Here's how the part is built. I have some questions about the finished solid (model axes, mm). Face numbers are marked on the shaded views. A direction names the side the tool comes from. Coordinates: 2 decimals unless noted, no trailing zeros. Write each loop counter-clockwise with the first axis right and the second up, starting at its lowest first coordinate (ties: lowest second). Pieces come first, ordered by that corner, then holes.
Item 1: If I drill on line 1 (X direction, y = -4.5, z = -3.75); line 2 (Y direction, x = -10, z = -9.5); line 3 (X direction, y = -2, z = -3.75), over which ranges is the centre line in solid material (lowest first)?
Item 2: If we section it at B-B (x = 0): Please give me the cut outline in (y, z).
Item 3: For the marked faces 5 and 6, which set-ups out of +Z, -Z, +X, -X, +Y, -Y let a thin tool reach every point of the face, with its end or its side?
Item 4: If we section it at A-A (z = -1): Please give me the cut outline in (x, y), then the cut area to 3 significant figures.
Item 5: I'm going to push flat-ended pins straight in: pin 1 Ø2.5 at (x, z) = (-6, -3) entering from +Y; pin 2 Ø4 at (x, y) = (0.03, -11.5) entering from -Z; pin 3 Ø5 at (x, y) = (-9.97, 5.73) entering from +Z; pin 4 Ø1.5 at (y, z) = (-4, -5) entering from -X. Where does each tip first touch, or does it pass through?
Item 6: If we section it at C-C (y = -11.5): Please give me the cut outline in (x, z).
Item 7: If we section it at D-D (x = 9): Please give me the cut outline in (y, z), then the cut area to 3 significant figures.
Item 8: We'd pull the mould along Y, two halves only. Please class the marked faces 1, 2, 3 and 4: +Y half, -Y half, draft (parallel to the pull), parting line (faces both ways), or undercut.
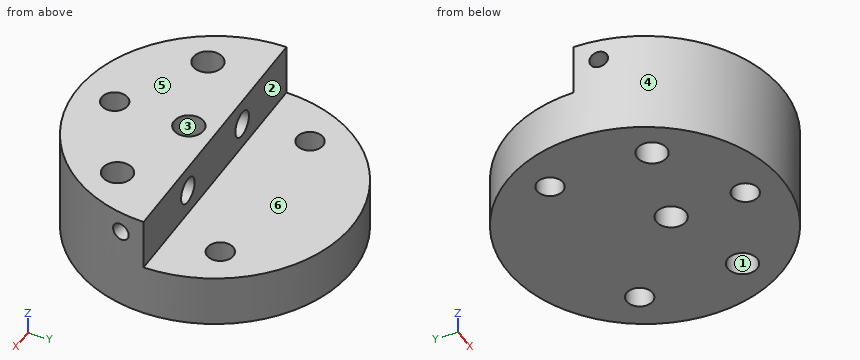
Autodesk Inventor part; units mm, degrees
ref_plane "作業平面8" through (15.56, -2.7436, 0) normal (0.9848, -0.1736, 0) x (0, 0, 1)
ref_plane "作業平面9" through (-15.56, -2.7436, 0) normal (0.9848, 0.1736, 0) x (0, 0, 1)
ref_plane "XZ Plane" through (0, 0, 0) normal (0, 1, 0) x (-1, 0, 0)
sketch "スケッチ2" plane through (0, 0, 0) normal (0, 0, 1) x (1, 0, 0)
  circle A0 centre (0, 0) radius 15.8
  dimension "d0" = 31.6
extrude "押し出し1" add sketch "スケッチ2" against normal blind 12
sketch "スケッチ4" plane through (0, 0, 0) normal (0, 0, 1) x (1, 0, 0)
  circle A0 centre (0.0258, -11.5) radius 1.5
  circle A1 centre (9.9464, 5.7723) radius 1.5
  circle A2 centre (-9.9722, 5.7277) radius 1.5
  point P0 (0, 0)
  dimension "d8" = 3
  dimension "d9" = 11.5
  dimension "d12" = 360
extrude "押し出し3" cut sketch "スケッチ4" against normal through all
sketch "スケッチ13" plane through (0, 0, 0) normal (0, 0, 1) x (1, 0, 0)
  circle A0 centre (-10, -6) radius 1.7
  circle A1 centre (10, -6) radius 1.7
  circle A2 centre (0, -3) radius 1.7
  line L0 (0, 0) -> (0, -19.4065)
  line L1 (0, 0) -> (20.4623, 0)
  point P0 (0, -4.7)
  point P1 (0, -1.3)
  dimension "d125" = 3.4
  dimension "d126" = 3.4
  dimension "d127" = 3.4
  dimension "d128" = 6
  dimension "d129" = 3
  dimension "d130" = 10
extrude "押し出し11" cut sketch "スケッチ13" against normal through all
ref_plane "作業平面6" through (0, 0, 0) normal (0.9848, -0.1736, 0) x (0, 0, 1)
ref_plane "作業平面7" through (0, 0, 0) normal (0.9848, 0.1736, 0) x (0, 0, 1)
ref_plane "作業平面8" through (15.56, -2.7436, 0) normal (0.9848, -0.1736, 0) x (0, 0, 1)
ref_plane "作業平面9" through (-15.56, -2.7436, 0) normal (0.9848, 0.1736, 0) x (0, 0, 1)
sketch "スケッチ15" plane through (15.56, -2.7436, 0) normal (0.9848, -0.1736, 0) x (0, 0, 1)
  circle A0 centre (-2.5, 0) radius 1
  point P0 (0, 0)
  dimension "d103" = 2
  dimension "d104" = 2.5
sketch "スケッチ16" plane through (-15.56, -2.7436, 0) normal (0.9848, 0.1736, 0) x (0, 0, 1)
  circle A0 centre (-2.5, 0) radius 1
  point P0 (0, 0)
  dimension "d105" = 2
  dimension "d106" = 2.5
extrude "押し出し12" cut sketch "スケッチ16" along normal blind 6
extrude "押し出し13" cut sketch "スケッチ15" against normal blind 6
thread "ねじ10"
thread "ねじ11"
sketch "スケッチ18" plane through (0, 0, 0) normal (0, 0, 1) x (1, 0, 0)
  line L0 (-18.9802, 17.2113) -> (19.0758, 17.2113)
  line L1 (19.0758, 17.2113) -> (19.0758, 0)
  line L2 (19.0758, 0) -> (-18.9802, 0)
  line L3 (-18.9802, 0) -> (-18.9802, 17.2113)
  point P0 (0, 0)
  point P1 (0.0478, 0)
  dimension "d141" = 0
extrude "押し出し15" cut sketch "スケッチ18" against normal blind 6
sketch "スケッチ20" plane through (-15.8, 0, 0) normal (0, 1, 0) x (1, 0, 0)
  line L0 (15.8, 0) -> (15.8, 8.7821) construction
  line L1 (0, 0) -> (0, 6)
  line L2 (0, 3) -> (33.9854, 3) construction
  circle A0 centre (9.8, 3) radius 1.5
  circle A1 centre (21.8, 3) radius 1.5
  line L3 (31.6, 0) -> (0, 0)
  dimension "d132" = 3
  dimension "d133" = 3
  dimension "d134" = 6
extrude "押し出し16" cut sketch "スケッチ20" against normal blind 8
thread "ねじ13"
thread "ねじ14"
thread "ねじ15"
thread "ねじ16"
thread "ねじ17"
properties part number "B_probehead_5_1" material "ステンレス鋼 440C"
Answer list:
1. line 1: x = -15.15 to -10.8, -9.2 to -7.3, -4.7 to -0.8, 0.8 to 4.7, 7.3 to 9.2, 10.8 to 15.15
1. line 2: y = -12.23 to -7.7, -4.3 to 4.23, 7.23 to 12.23
1. line 3: x = -15.67 to -7.3, -4.7 to -1.37, 1.37 to 4.7, 7.3 to 15.67
2. outline: (-15.8, -12) - (-13, -12) - (-13, 0) - (-15.8, 0) - close; (-10, -12) - (-4.7, -12) - (-4.7, 0) - (-10, 0) - close; (-1.3, -12) - (15.8, -12) - (15.8, -6) - (0, -6) - (0, 0) - (-1.3, 0) - close
3. face 5: +Z, +X, -X, +Y, -Y
3. face 6: +Z, +X, -X, +Y
4. outline: (-15.8, 0) arc R15.8 ccw to (15.8, 0) - close; hole circle Ø3.4 at (-10, -6); hole circle Ø3.4 at (0, -3); hole circle Ø3 at (0.03, -11.5); hole circle Ø3.4 at (10, -6)
4. area: 358 mm2
5. pin 1: stops at y = -8
5. pin 2: stops at z = -12
5. pin 3: stops at z = -6
5. pin 4: stops at x = -15.46
6. outline: (-10.83, -12) - (-1.47, -12) - (-1.47, 0) - (-10.83, 0) - close; (1.53, -12) - (10.83, -12) - (10.83, 0) - (1.53, 0) - close
7. outline: (-12.99, -12) - (-7.37, -12) - (-7.37, 0) - (-12.99, 0) - close; (-4.63, -12) - (4.61, -12) - (4.61, -6) - (0, -6) - (0, 0) - (-4.63, 0) - close; (6.94, -12) - (12.99, -12) - (12.99, -6) - (6.94, -6) - close
7. area: 187 mm2
8. face 1: undercut
8. face 2: +Y half
8. face 3: undercut
8. face 4: parting line
